Geometry: final body of the model. Coordinates: model frame, mm. A direction names the side the tool comes from. Give positions to 0.01 mm unless a question says otherwise; leave off trailing zeros. Write each loop counter-clockwise with the first axis right and the second up, starting at its lowest first coordinate (ties: lowest second). Pieces come first, ordered by that corner, then holes.
Q1. Draft query along Z for faces 3 (the face through (100.18, 18.1, -18.14)), 4 (the face through (100, 19.05, 0)), 5 (the face through (100, 0, -15.875)), 6 (the face through (100.18, -14.97, 14.92)). Return one class per face: pulls with the +Z half, pulls with the -Z half, needs draft (parallel to the pull), parting line crosses it, or undercut.
Q2. Cut plane A-A on y = -4.5. Return the cut outline in (x, z) (3 decimals), plus the area to 3 significant figures.
Q3. Pin query (flat end, axial travel): pin 1 (8 mm diameter, centred on y = 3, z = -12, fed in from +X). Return the tip coordinate at first contact, or that it passes through.
Q4. Reachability of faces 1 (the face through (100.18, 14.92, 14.97)), 2 (the face through (100, 0, -19.05)) from +Z, -Z, +X, -X, +Y, -Y: full face, straight path, thin tool, end or side. Return the list, or none.
Q5. Line query: L1, parallel to Z at x = 21, y = 11 (3 decimals); L2, parallel to Z at x = 98, y = -16. Output: solid intervals per line, ascending.
Q6. Cut plane B-B on x = 166. Return the cut outline in (y, z) (3 decimals), plus the area to 3 significant figures.
```python
from build123d import *

# Parameters (mm, degrees)
F1_DEPTH = 203.2


with BuildPart() as f1:
    # F0 (on Right) → F1 (new body)
    with BuildSketch(Plane.YZ):
        with BuildLine():
            ThreePointArc((19.05, 15.875), (18.120064, 18.120064), (15.875, 19.05))
            Line((15.875, 19.05), (-15.875, 19.05))
            ThreePointArc((-15.875, 19.05), (-18.120064, 18.120064), (-19.05, 15.875))
            Line((-19.05, 15.875), (-19.05, -15.875))
            ThreePointArc((-19.05, -15.875), (-18.120064, -18.120064), (-15.875, -19.05))
            Line((-15.875, -19.05), (15.875, -19.05))
            ThreePointArc((15.875, -19.05), (18.120064, -18.120064), (19.05, -15.875))
            Line((19.05, -15.875), (19.05, 15.875))
        make_face()
        with BuildLine():
            Line((-12.7, 15.875), (12.7, 15.875))
            ThreePointArc((12.7, 15.875), (14.945064, 14.945064), (15.875, 12.7))
            Line((15.875, 12.7), (15.875, -12.7))
            ThreePointArc((15.875, -12.7), (14.945064, -14.945064), (12.7, -15.875))
            Line((12.7, -15.875), (-12.7, -15.875))
            ThreePointArc((-12.7, -15.875), (-14.945064, -14.945064), (-15.875, -12.7))
            Line((-15.875, -12.7), (-15.875, 12.7))
            ThreePointArc((-15.875, 12.7), (-14.945064, 14.945064), (-12.7, 15.875))
        make_face(mode=Mode.SUBTRACT)
    extrude(amount=F1_DEPTH)


solid = f1.part
```
Data:
1. face 3: pulls with the -Z half
1. face 4: needs draft
1. face 5: undercut
1. face 6: undercut
2. outline: (0, -19.05) - (203.2, -19.05) - (203.2, -15.875) - (0, -15.875) - close; (0, 15.875) - (203.2, 15.875) - (203.2, 19.05) - (0, 19.05) - close
2. area: 1,290 mm2
3. pin 1: stops at x = 203.2
4. face 1: +X, -X
4. face 2: -Z, +X, -X, +Y, -Y
5. L1: z = -19.05 to -15.875, 15.875 to 19.05
5. L2: z = -19.05 to 19.05
6. outline: (-19.05, -15.875) arc R3.175 ccw to (-15.875, -19.05) - (15.875, -19.05) arc R3.175 ccw to (19.05, -15.875) - (19.05, 15.875) arc R3.175 ccw to (15.875, 19.05) - (-15.875, 19.05) arc R3.175 ccw to (-19.05, 15.875) - close; hole (-15.875, -12.7) arc R3.175 ccw to (-12.7, -15.875) - (12.7, -15.875) arc R3.175 ccw to (15.875, -12.7) - (15.875, 12.7) arc R3.175 ccw to (12.7, 15.875) - (-12.7, 15.875) arc R3.175 ccw to (-15.875, 12.7) - close
6. area: 444 mm2
